```python
from build123d import *

# Parameters (mm, degrees)
SKETCH_W        = 100
SKETCH_H        = 52
SKETCH_R        = 1.25
SKETCH_R_2      = 9.25
PAD_DEPTH       = 4
SKETCH001_W     = 4
SKETCH001_H     = 52
PAD001_DEPTH    = 5
SKETCH002_W     = 82
SKETCH002_H     = 1.5
POCKET_DEPTH    = 2
SKETCH003_R     = 2.05
POCKET001_DEPTH = 5
FILLET_R        = 1
FILLET001_R     = 1
SKETCH004_W     = 4
SKETCH004_H     = 1.5
POCKET002_DEPTH = 2


with BuildPart() as part:
    # Sketch → Pad (new body)
    with BuildSketch(Plane.XY):
        with Locations((0, 5)):
            Rectangle(SKETCH_W, SKETCH_H)
        with Locations((13.5, 11)):
            Circle(SKETCH_R, mode=Mode.SUBTRACT)
        with Locations((13.5, -11)):
            Circle(SKETCH_R, mode=Mode.SUBTRACT)
        with Locations((13.5, -17)):
            Circle(SKETCH_R, mode=Mode.SUBTRACT)
        with Locations((45, -17)):
            Circle(SKETCH_R, mode=Mode.SUBTRACT)
        with Locations((45, 11)):
            Circle(SKETCH_R, mode=Mode.SUBTRACT)
        with Locations((-6.5, 11)):
            Circle(SKETCH_R_2, mode=Mode.SUBTRACT)
        with BuildLine():
            Line((46, 3), (46, -3))
            ThreePointArc((44, -3), (45, -4), (46, -3))
            Line((44, -3), (44, 3))
            ThreePointArc((46, 3), (45, 4), (44, 3))
        make_face(mode=Mode.SUBTRACT)
        with BuildLine():
            Line((14.5, 3), (14.5, -3))
            ThreePointArc((12.5, -3), (13.5, -4), (14.5, -3))
            Line((12.5, 3), (12.5, -3))
            ThreePointArc((14.5, 3), (13.5, 4), (12.5, 3))
        make_face(mode=Mode.SUBTRACT)
    extrude(amount=PAD_DEPTH)

    # Sketch001 (on Face20 of Pad) → Pad001 (join)
    with BuildSketch(Plane.XY.offset(4)):
        with Locations((-48, 5)):
            Rectangle(SKETCH001_W, SKETCH001_H)
        with Locations((30, 5)):
            Rectangle(SKETCH001_W, SKETCH001_H)
    extrude(amount=PAD001_DEPTH)

    # Sketch002 (on Face26 of Pad001) → Pocket (cut)
    with BuildSketch(Plane.XY.offset(9)):
        with Locations((-9, 28.25)):
            Rectangle(SKETCH002_W, SKETCH002_H)
        with Locations((-9, 23.25)):
            Rectangle(SKETCH002_W, SKETCH002_H)
        with Locations((-9, -17)):
            Rectangle(SKETCH002_W, SKETCH002_H)
    extrude(amount=-POCKET_DEPTH, mode=Mode.SUBTRACT)

    # Sketch003 (on Face6 of Pocket) → Pocket001 (cut)
    with BuildSketch(Plane.XY.offset(4)):
        with Locations((-40, 25)):
            Circle(SKETCH003_R)
        with Locations((-40, -16)):
            Circle(SKETCH003_R)
        with Locations((22, 25)):
            Circle(SKETCH003_R)
        with Locations((22, -16)):
            Circle(SKETCH003_R)
    extrude(amount=-POCKET001_DEPTH, mode=Mode.SUBTRACT)

    # Fillet
    fillet_edges = [part.edges().sort_by_distance(p)[0] for p in [
        (-50, -21, 2),
        (50, -21, 2),
        (50, 31, 2),
        (-50, 31, 2),
    ]]
    fillet(fillet_edges, radius=FILLET_R)

    # Fillet001
    fillet001_edges = [part.edges().sort_by_distance(p)[0] for p in [
        (-46, 31, 6.5),
        (-46, -21, 6.5),
        (28, 31, 6.5),
        (32, 31, 6.5),
        (28, -21, 6.5),
        (32, -21, 6.5),
    ]]
    fillet(fillet001_edges, radius=FILLET001_R)

    # Sketch004 (on Face41 of Fillet001) → Pocket002 (cut)
    with BuildSketch(Plane.XY.offset(9)):
        with Locations((-48, 11)):
            Rectangle(SKETCH004_W, SKETCH004_H)
    extrude(amount=-POCKET002_DEPTH, mode=Mode.SUBTRACT)


solid = part.part
```
Source: CAD feature listing. Evaluate the final solid. Frame: model axes, mm. A direction names the side the tool comes from. Give positions to 0.01 mm unless a question says otherwise; leave off trailing zeros. Write each loop counter-clockwise with the first axis right and the second up, starting at its lowest first coordinate (ties: lowest second). Pieces come first, ordered by that corner, then holes. Notation, with made-up numbers: (82.5, -22.5) - (140.5, -22.5) arc R19 ccw to (140.5, 12.5) - close; hole circle Ø10 at (-14.75, -15). An arc over 180 degrees is marked (long way). One line per item, written item: value. Start each with the question number.
Q1. Section query A-A, the plane x = -6.5. Return the cut outline in (y, z).
Q2. Section query D-D, the plane y = -2. Return the cut outline in (x, z).
Q3. Section query C-C, the plane z = 6. Return the cut outline in (x, y).
Q4. Draft query along Y for faces 4 (the face through (40, 5, 4)), 5 (the face through (-48, 10.25, 8)). Return one class per face: +Y half, -Y half, draft (parallel to the pull), parting line (faces both ways), or undercut.
Q5. Set-up query: faces 1 (the face through (13.5, -4, 2)), 2 (the face through (-48, -19, 9)), 3 (the face through (30, 24, 8)). Return all of +Z, -Z, +X, -X, +Y, -Y with unobstructed straight access to the full face (end or side cutting, diameter ignored); none if empty.
Q6. First-contact query: pin 1 Ø4.5 at (x, y) = (-40, 25) entering from -Z; pin 2 Ø10 at (x, y) = (-15.5, 9.5) entering from +Z; pin 3 Ø1 at (y, z) = (-9, 7) entering from +X. Flat tips, straight axial feed; report the tip coordinate or a pass-through.
Q7. Section query B-B, the plane x = 13.5. Return the cut outline in (y, z).
Q8. Material intervals for probe 1 along Y at (x, z) = (13.5, 1.75); probe 2 along Y at (x, z) = (45, 1.4); probe 3 along Y at (x, z) = (22, 1), sorted ascending. Write a range as from..to.
Answer:
1. outline: (-21, 0) - (1.75, 0) - (1.75, 4) - (-21, 4) - close; (20.25, 0) - (31, 0) - (31, 4) - (20.25, 4) - close
2. outline: (-50, 0) - (12.5, 0) - (12.5, 4) - (-46, 4) - (-46, 9) - (-50, 9) - close; (14.5, 0) - (44, 0) - (44, 4) - (32, 4) - (32, 9) - (28, 9) - (28, 4) - (14.5, 4) - close; (46, 0) - (50, 0) - (50, 4) - (46, 4) - close
3. outline: (-50, -20) arc R1 ccw to (-49, -21) - (-47, -21) arc R1 ccw to (-46, -20) - (-46, 30) arc R1 ccw to (-47, 31) - (-49, 31) arc R1 ccw to (-50, 30) - close; (28, -20) arc R1 ccw to (29, -21) - (31, -21) arc R1 ccw to (32, -20) - (32, 30) arc R1 ccw to (31, 31) - (29, 31) arc R1 ccw to (28, 30) - close
4. face 4: draft
4. face 5: undercut
5. face 1: +Z, -Z
5. face 2: +Z, +X, -X, +Y, -Y
5. face 3: +Z, +X, -X
6. pin 1: stops at z = 0
6. pin 2: stops at z = 4
6. pin 3: stops at x = 32
7. outline: (-21, 0) - (-18.25, 0) - (-18.25, 4) - (-21, 4) - close; (-15.75, 0) - (-12.25, 0) - (-12.25, 4) - (-15.75, 4) - close; (-9.75, 0) - (-4, 0) - (-4, 4) - (-9.75, 4) - close; (4, 0) - (9.75, 0) - (9.75, 4) - (4, 4) - close; (12.25, 0) - (31, 0) - (31, 4) - (12.25, 4) - close
8. probe 1: y = -21..-18.25, -15.75..-12.25, -9.75..-4, 4..9.75, 12.25..31
8. probe 2: y = -21..-18.25, -15.75..-4, 4..9.75, 12.25..31
8. probe 3: y = -21..-18.05, -13.95..22.95, 27.05..31
